from build123d import *

# Parameters (mm, degrees)
SKETCH1_W           = 31.5
SKETCH1_H           = 44
BOSS_EXTRUDE1_DEPTH = 1.5
SKETCH2_W           = 11.18
SKETCH2_H           = 2.54
BOSS_EXTRUDE2_DEPTH = 3.81
SKETCH4_W           = 11.18
SKETCH4_H           = 1.746
CUT_EXTRUDE1_DEPTH  = 3.81
SKETCH5_W           = 21.34
SKETCH5_H           = 2.54
BOSS_EXTRUDE3_DEPTH = 3.81
SKETCH8_W           = 21.34
SKETCH8_H           = 2.032
BOSS_EXTRUDE4_DEPTH = 2.032


with BuildPart() as part:
    # Sketch1 → Boss-Extrude1 (new body)
    with BuildSketch(Plane.XY):
        with Locations((13.046077502, 22)):
            Rectangle(SKETCH1_W, SKETCH1_H)
    extrude(amount=BOSS_EXTRUDE1_DEPTH)

    # Sketch2 → Boss-Extrude2 (add)
    with BuildSketch(Plane.XY.offset(1.5)):
        with Locations((13.046077502, 40.73)):
            Rectangle(SKETCH2_W, SKETCH2_H)
    extrude(amount=BOSS_EXTRUDE2_DEPTH)

    # Sketch4 → Cut-Extrude1 (cut)
    with BuildSketch(Plane.XY.offset(1.5)):
        with Locations((13.046077502, 43.127)):
            Rectangle(SKETCH4_W, SKETCH4_H)
    extrude(amount=-CUT_EXTRUDE1_DEPTH, mode=Mode.SUBTRACT)

    # Sketch5 → Boss-Extrude3 (add)
    with BuildSketch(Plane.XY.offset(1.5)):
        with Locations((13.046077502, 1.27)):
            Rectangle(SKETCH5_W, SKETCH5_H)
    extrude(amount=BOSS_EXTRUDE3_DEPTH)

    # Sketch8 → Boss-Extrude4 (add)
    with BuildSketch(Plane(origin=(0, 0, 0), x_dir=(-1, 0, 0), z_dir=(0, -1, 0))):
        with Locations((-13.046077502, -4.294)):
            Rectangle(SKETCH8_W, SKETCH8_H)
    extrude(amount=BOSS_EXTRUDE4_DEPTH)


solid = part.part
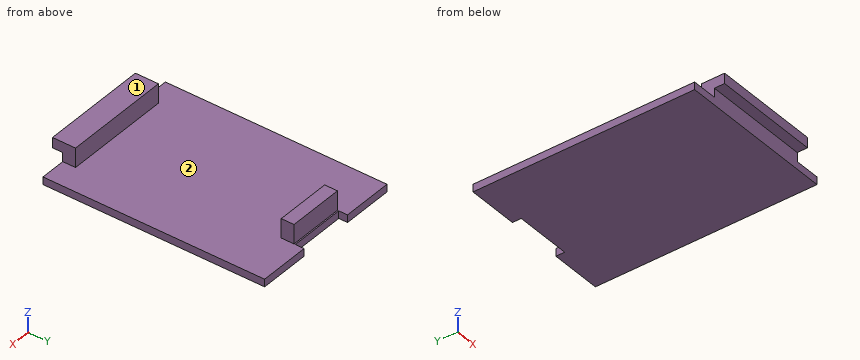
Can you work these out from the model? Positions are in its coordinate system, mm. Face numbers are marked on the shaded views. Give positions to 0.01 mm unless a question says otherwise; leave off trailing zeros. Order: outer loops, then holes, each group sorted by start corner. A loop starts at its lowest first (then second) coordinate and runs counter-clockwise, first axis right, second up. Notation, with made-up numbers: M -9,23.25 L 28,23.25 A16 ccw 28,43.25 Z; hole C 58,37 d9. An arc over 180 degrees is marked long. One line per item, written item: value.
Item 1: If we section it at C-C on y = 35: Write out the boundary of the cut face in (x, z).
Verdict:
outline: M -2.7,0 L 28.8,0 L 28.8,1.5 L -2.7,1.5 Z
Item 2: If we section it at A-A on z = 2.55: Write out the boundary of the cut face in (x, y), and give its area (3 significant figures).
Verdict:
outline: M 2.38,0 L 23.72,0 L 23.72,2.54 L 2.38,2.54 Z; M 7.46,39.46 L 18.64,39.46 L 18.64,42 L 7.46,42 Z
area: 82.6 mm2
Item 3: If we mould it in two halves opening along Y, with no side actions, what happens to the marked faces 1 and 2? For each: pulls with the +Y half, pulls with the -Y half, needs draft (parallel to the pull), parting line crosses it, or undercut.
Verdict:
face 1: needs draft
face 2: undercut
Item 4: If we section it at D-D on x = 9: Write out the boundary of the cut face in (y, z).
Verdict:
outline: M -2.03,3.28 L 0,3.28 L 0,0 L 42.25,0 L 42.25,1.5 L 42,1.5 L 42,5.31 L 39.46,5.31 L 39.46,1.5 L 2.54,1.5 L 2.54,5.31 L -2.03,5.31 Z
Item 5: Please list where these lines run through material, in increasing order: line 1 (Y direction, x = 14.5, z = 4.5); line 2 (Y direction, x = 16, z = 1.95); line 3 (Z direction, x = 11.5, y = 12).
Verdict:
line 1: -2.03 to 2.54, 39.46 to 42
line 2: 0 to 2.54, 39.46 to 42
line 3: 0 to 1.5
Item 6: If we section it at B-B on x = 5.5: Write out the boundary of the cut face in (y, z).
Verdict:
outline: M -2.03,3.28 L 0,3.28 L 0,0 L 44,0 L 44,1.5 L 2.54,1.5 L 2.54,5.31 L -2.03,5.31 Z
Item 7: For pin 1 (3 mm diameter, centred on x = 23.5, z = 2.5, fed in from +Y); pin 2 (1.9 mm diameter, centred on y = 0.5, z = 4, fed in from -X); pin 3 (3 mm diameter, centred on x = 12, z = 3.5, fed in from +Y); pin 4 (1.5 mm diameter, centred on y = 8, z = 3, fed in from +X), each with a flat end and sliding along its axis, tell me the tip position at first contact or that it passes through.
Verdict:
pin 1: y = 44
pin 2: x = 2.38
pin 3: y = 42
pin 4: through
